Solid Edge part; units mm, degrees
sketch "Sketch1" plane through (0, 0, 0) normal (0, 0, 1) x (1, 0, 0)
  line L0 (-110, -40) -> (110, -40)
  line L1 (110, -40) -> (110, 40)
  line L2 (110, 40) -> (-110, 40)
  line L3 (-110, 40) -> (-110, -40)
  dimension "D1" = 110
  dimension "D2" = 110
extrude "Protrusion1" add sketch "Sketch1" along normal blind 10
sketch "Sketch2" plane through (0, 0, 10) normal (0, 0, 1) x (1, 0, 0)
  circle A0 centre (15, -30) radius 5
extrude "Cutout1" cut sketch "Sketch2" against normal through all
sketch "Sketch3" plane through (0, 0, 10) normal (0, 0, 1) x (1, 0, 0)
  circle A0 centre (-15, -20) radius 4.5
  circle A1 centre (-36.92, -20) radius 1.6
  circle A2 centre (6.92, -20) radius 1.6
extrude "Cutout2" cut sketch "Sketch3" against normal up to next
sketch "Sketch4" plane through (0, -40, 5) normal (0, -1, 0) x (1, 0, 0)
  line L0 (-110, 5) -> (110, 5)
  line L1 (110, 5) -> (110, -5)
  line L2 (110, -5) -> (-110, -5)
  line L3 (-110, -5) -> (-110, 5)
extrude "Extrusionsausprägung_2" add sketch "Sketch4" along normal blind 10
sketch "Sketch5" plane through (0, -5, 10) normal (0, 0, 1) x (1, 0, 0)
  circle A0 centre (-90, -25) radius 5
  dimension "D1" = 90
extrude "Cutout3" cut sketch "Sketch5" against normal up to next
hole "Bohrung_1" at (-90, -41, 10) direction (0, 0, -1) diameter 3.2 end up to next
hole "Hole1" at (-101, -30, 10) direction (0, 0, -1) diameter 3.2 end up to next
hole "Hole2" at (-79, -30, 10) direction (0, 0, -1) diameter 3.2 end up to next
hole "Hole3" at (-90, -19, 10) direction (0, 0, -1) diameter 3.2 end up to next
mirror "Mirror1" about plane through (0, 0, 0) normal (1, 0, 0) of "Cutout3", "Bohrung_1", "Hole1", "Hole2", "Hole3"
properties material "Nylon, allgemein"
Geometry check sheet. Reference: the model listing, model coordinates, mm. Round coordinates to 2 decimals unless told otherwise and drop trailing zeros. Order: outer loops, then holes, each group sorted by start corner. A loop starts at its lowest first (then second) coordinate and runs counter-clockwise, first axis right, second up. Notation, with made-up numbers: M -28.75,-4.5 L -2.75,-4.5 A16 cw -2.75,10.5 Z; hole C 31,82 d5. An arc over 180 degrees is marked long. Write item = value, one per line.
Q1. Release check for a two-part mould opening along X. For faces 1 (the cylindrical face through (19.619, -31.915, 5.07)), 2 (the flat face through (-2, -4, 10)), 3 (the flat face through (-110, -4, 5)), 4 (the cylindrical face through (85.381, -28.085, 5.07)) record: released by +X, released by -X, zero draft, split by the parting line, or undercut.
Answer block:
face_1 = undercut
face_2 = zero draft
face_3 = released by -X
face_4 = undercut
Q2. Depth check by flat-ended pin: pin 1 Ø2.5 at (x, y) = (-79, -30) entering from -Z. Enter the tip coordinate at first touch or a pass-through.
Answer block:
pin_1 = through
Q3. Section check B-B (z = 7.5). Give the number of separate pieces and of enclosed holes in the cut face, plus the area to 3 significant figures.
Answer block:
separate_pieces = 1
enclosed_holes = 14
area = 19,400 mm^2
Q4. Section check A-A (x = -15). Enter the section's corners in (y, z).
Answer block:
outline = M -50,0 L -24.5,0 L -24.5,10 L -50,10 Z; M -15.5,0 L 40,0 L 40,10 L -15.5,10 Z
Q5. Section check C-C (x = 13.5). Enter the section's corners in (y, z), plus the area to 3 significant figures.
Answer block:
outline = M -50,0 L -34.77,0 L -34.77,10 L -50,10 Z; M -25.23,0 L 40,0 L 40,10 L -25.23,10 Z
area = 805 mm^2
Q6. Scan lines: line 1 (Y direction, x = -90, z = 2.5); line 2 (X direction, y = -41, z = 4.25); line 3 (Y direction, x = 79, z = 5.5). Record each from-to range of solid material in increasing order.
Answer block:
line_1 = -50 to -42.6, -39.4 to -35, -25 to -20.6, -17.4 to 40
line_2 = -110 to -91.6, -88.4 to 88.4, 91.6 to 110
line_3 = -50 to -31.6, -28.4 to 40
